Read the model definition and answer for the solid it produces. Units are mm, in the model's axes. Give positions to 0.01 mm unless a question says otherwise; leave off trailing zeros. Write each loop counter-clockwise with the first axis right and the second up, starting at its lowest first coordinate (ties: lowest second). Pieces come first, ordered by that corner, then holes. Notation, with made-up numbers: (38.25, -22.75) -> (69.25, -22.75) arc R28 ccw to (69.25, -4.75) -> close; hole circle Ø3 at (62.5, 47). An arc over 180 degrees is marked (long way). Use a Markdown table: item, result.
Autodesk Fusion 360 part; units mm, degrees
sketch "Sketch1" plane through (0, 0, 0) normal (0, 0, 1) x (1, 0, 0)
  line L0 (0, 0) -> (40, 0) construction
  line L1 (0, 10) -> (40, 10)
  line L2 (0, -10) -> (40, -10)
  arc A0 (0, 10) -> (0, -10) centre (0, 0) ccw
  arc A1 (40, -10) -> (40, 10) centre (40, 0) ccw
  circle A2 centre (45, 0) radius 1.75
  line L3 (50, 9.724) -> (50, -11.0876) construction
  dimension "d1" = 20
  dimension "d2" = 20
  dimension "d3" = 40
  dimension "d4" = 3.5
  dimension "d5" = 5
extrude "Extrude1" add sketch "Sketch1" along normal blind 3
sketch "DXF_outline" plane through (0, 0, 3) normal (0, 0, 1) x (-1, 0, 0)
  circle A0 centre (-45, 0) radius 1.75
  arc A1 (0, -10) -> (0, 10) centre (0, 0) ccw
  line L0 (0, 10) -> (-40, 10)
  arc A2 (-40, 10) -> (-40, -10) centre (-40, 0) ccw
  line L1 (-40, -10) -> (0, -10)
equation "d1 = width"
equation "d2 = d1"
equation "d3 = length"
equation "d4 = keyhole"
equation "d5 = d4 + 1.5 mm"
equation "width = 20 mm"
equation "length = 40 mm"
equation "keyhole = 3.5 mm"
Item 1: A cutting plane is placed at A-A (x = 46). Give the vertices of the cut face in (y, z).
Return value:
| item | result |
|---|---|
| outline | (-8, 0) -> (-1.44, 0) -> (-1.44, 3) -> (-8, 3) -> close; (1.44, 0) -> (8, 0) -> (8, 3) -> (1.44, 3) -> close |
Item 2: A cutting plane is placed at D-D (x = -3). Give the vertices of the cut face in (y, z).
Return value:
| item | result |
|---|---|
| outline | (-9.54, 0) -> (9.54, 0) -> (9.54, 3) -> (-9.54, 3) -> close |
Item 3: Straight lines are drawn through the part: line 1 along Y through (x, z) = (40.5, 1.2); line 2 along X through (y, z) = (-1.25, 1.5); line 3 along X through (y, z) = (-0.75, 1.3). For each, find the intervals that lie inside material, in ascending order. Write a range as [from, to].
Return value:
| item | result |
|---|---|
| line 1 | [-9.99, 9.99] |
| line 2 | [-9.92, 43.78], [46.22, 49.92] |
| line 3 | [-9.97, 43.42], [46.58, 49.97] |
Item 4: For a pull along Y with two mould halves and no side action, classify faces 1 (the face through (46.617, 0.67, 1.479)), 2 (the face through (50, 0, 1)), 3 (the face through (20, -10, 1)) as +Y half, -Y half, draft (parallel to the pull), parting line (faces both ways), or undercut.
Return value:
| item | result |
|---|---|
| face 1 | undercut |
| face 2 | parting line |
| face 3 | -Y half |
Item 5: This flat-tipped pin is pushed along its axis until it touches: P1, Ø1.5, axis at y = -5, z = 1, coming from the -X side. Where does it stop, or does it pass through?
Return value:
| item | result |
|---|---|
| P1 | x = -9.05 |
Item 6: A cutting plane is placed at B-B (z = 0.75). Give the vertices of the cut face in (x, y).
Return value:
| item | result |
|---|---|
| outline | (0, -10) -> (40, -10) arc R10 ccw to (40, 10) -> (0, 10) arc R10 ccw to start; hole circle Ø3.5 at (45, 0) |
Item 7: A cutting plane is placed at C-C (y = 4). Give the vertices of the cut face in (x, z).
Return value:
| item | result |
|---|---|
| outline | (-9.17, 0) -> (49.17, 0) -> (49.17, 3) -> (-9.17, 3) -> close |
